The drawing under review shows one solid part. Ordinate dimensions are in mm from its lowest x, y, z. A direction names the side the tool comes from. Give positions to 0.01 mm unless a question says otherwise; leave off trailing zeros. Loops run counter-clockwise (first coordinate to the right, second up) from the corner with the lowest first, then second, coordinate; pieces in that order, holes last. Notation, with made-up numbers: M -10.5,-20 L -1.5,-20 A12 ccw -1.5,-1 Z; hole C 67,-16.75 d11. An arc over 180 degrees is marked long. Put each result on its own line as item: value. Start each with the question number.
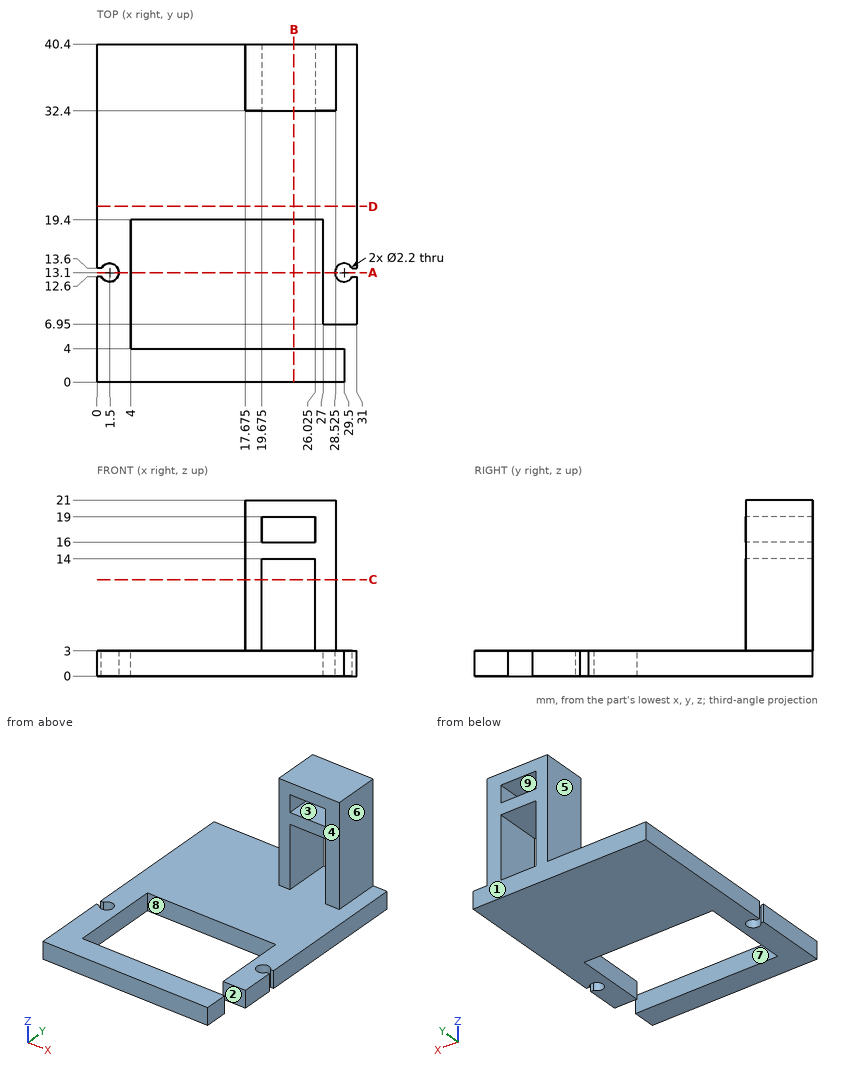
(1) We need section B-B, the plane x = 23.5. Write out the cut boundary in (y, z), plus the area to 3 significant figures.
(2) We need section A-A, the plane y = 13.1. Write out the cut boundary in (x, z).
(3) To check wall thickness, follow L1, parallel to Z at x = 21.5, y = 33; L2, parallel to X at y = 13.1, z = 0.95; L3, parallel to Y at x = 8, z = 2. State the ranges of each line that lie inside material, in increasing order. Write a range as [from, to].
(4) For the marked faces 5, 6, 7, 8 and 9, list the 3-axis set-ups (+Z, -Z, +X, -X, +Y, -Y) from which the entire face can be reached by the end or side of a thin tool; tool diameter is ignored.
(5) We need section C-C, the plane z = 11.5. Write out the cut boundary in (x, y) (3 decimals), plus the area to 3 significant figures.
(6) We need section D-D, the plane y = 21. Write out the cut boundary in (x, z).
(7) Insertion check: pin 1 (4 mm diameter, centred on y = 37.5, z = 13, fed in from -X) (3 decimals); pin 2 (4 mm diameter, centred on x = 21, z = 18.5, fed in from -Y); pin 3 (1.5 mm diameter, centred on y = 34.5, z = 17.5, fed in from +X) (3 decimals). Each pin has a flat end and moves straight along its axis. Give the tip position at first contact, or say it passes through.
(8) Draft analysis for pull direction Y (two halves, no side actions). For the marked faces 1, 2, 3 and 4, state which applies: +Y half, -Y half, draft (parallel to the pull), parting line (faces both ways), or undercut.
Check sheet entries:
1. outline: M 0,0 L 4,0 L 4,3 L 0,3 Z; M 19.4,0 L 40.4,0 L 40.4,3 L 19.4,3 Z; M 32.4,14 L 40.4,14 L 40.4,16 L 32.4,16 Z; M 32.4,19 L 40.4,19 L 40.4,21 L 32.4,21 Z
1. area: 107 mm²
2. outline: M 2.6,0 L 4,0 L 4,3 L 2.6,3 Z; M 27,0 L 28.4,0 L 28.4,3 L 27,3 Z
3. L1: z = [0, 3], [14, 16], [19, 21]
3. L2: x = [2.6, 4], [27, 28.4]
3. L3: y = [0, 4], [19.4, 40.4]
4. face 5: +Z, -X, +Y, -Y
4. face 6: +Z, +X, +Y, -Y
4. face 7: +Z, -Z, +X
4. face 8: +Z, -Z
4. face 9: +Y, -Y
5. outline: M 17.675,32.4 L 19.675,32.4 L 19.675,40.4 L 17.675,40.4 Z; M 26.025,32.4 L 28.525,32.4 L 28.525,40.4 L 26.025,40.4 Z
5. area: 36.0 mm²
6. outline: M 0,0 L 31,0 L 31,3 L 0,3 Z
7. pin 1: stops at x = 17.675
7. pin 2: stops at y = 32.4
7. pin 3: stops at x = 28.525
8. face 1: +Y half
8. face 2: undercut
8. face 3: draft
8. face 4: -Y half
